```python
from build123d import *

# Parameters (mm, degrees)
SKETCH001_R       = 0.35
PAD001_DEPTH      = 13.5
PAD001_DEPTH_BACK = 3.5
SKETCH_R          = 9
PAD_DEPTH         = 27
FILLET_R          = 0.5


with BuildPart() as pad001:
    # Sketch001 → Pad001 (new body, two sides)
    with BuildSketch(Plane.XY.offset(0.5)) as pad001_sk:
        Circle(SKETCH001_R)
        with Locations((10, 0)):
            Circle(SKETCH001_R)
    extrude(amount=PAD001_DEPTH)
    extrude(pad001_sk.sketch, amount=-PAD001_DEPTH_BACK)


with BuildPart() as l_radial_d18_0mm_p10_00mm:
    # Sketch → Pad (new body)
    with BuildSketch(Plane.XY.offset(0.1)):
        with Locations((5, 0)):
            Circle(SKETCH_R)
    extrude(amount=PAD_DEPTH)

    # Fillet
    fillet_edges = [l_radial_d18_0mm_p10_00mm.edges().sort_by_distance(p)[0] for p in [
        (-4, 0, 0.1),
        (-4, 0, 27.1),
    ]]
    fillet(fillet_edges, radius=FILLET_R)

    add(pad001.part)


solid = l_radial_d18_0mm_p10_00mm.part
```
CAD build for the part. Positions are in the model's coordinates, mm. Give positions to 0.01 mm unless a question says otherwise; leave off trailing zeros. Order: outer loops, then holes, each group sorted by start corner. A loop starts at its lowest first (then second) coordinate and runs counter-clockwise, first axis right, second up.
(1) Saw through at A-A, the plane x = 5. Give the cut face in (y, z), then the cut area to 3 significant figures.
(2) Drill centre lines: L1, parallel to Z at x = 7.75, y = -7.5; L2, parallel to Y at x = 5, z = 5.5; L3, parallel to Y at x = 7.5, z = 14.5. Where is each one in solid material? Low to high.
(3) Flat gauge pins, fed straight in: pin 1 (3 mm diameter, centred on x = 0.5, z = 21, fed in from -Y); pin 2 (2 mm diameter, centred on x = 8.5, z = 24, fed in from +Y); pin 3 (8 mm diameter, centred on x = 2.5, y = -4.5, fed in from -Z). Where does each tip first touch, or does it go through?
(4) Saw through at C-C, the plane z = 6.5. Give the cut face in (x, y).
(5) Saw through at B-B, the plane y = 0. Give the cut face in (x, z).
Results found:
1. outline: (-9, 0.6) arc R0.5 ccw to (-8.5, 0.1) - (8.5, 0.1) arc R0.5 ccw to (9, 0.6) - (9, 26.6) arc R0.5 ccw to (8.5, 27.1) - (-8.5, 27.1) arc R0.5 ccw to (-9, 26.6) - close
1. area: 486 mm2
2. L1: z = 0.1 to 27.1
2. L2: y = -9 to 9
2. L3: y = -8.65 to 8.65
3. pin 1: stops at y = -8.49
3. pin 2: stops at y = 8.65
3. pin 3: stops at z = 0.1
4. outline: circle Ø18 at (5, 0)
5. outline: (-4, 0.6) arc R0.5 ccw to (-3.5, 0.1) - (-0.35, 0.1) - (-0.35, -3) - (0.35, -3) - (0.35, 0.1) - (9.65, 0.1) - (9.65, -3) - (10.35, -3) - (10.35, 0.1) - (13.5, 0.1) arc R0.5 ccw to (14, 0.6) - (14, 26.6) arc R0.5 ccw to (13.5, 27.1) - (-3.5, 27.1) arc R0.5 ccw to (-4, 26.6) - close
